from build123d import *

# Parameters (mm, degrees)
IZIM1_W                     = 15
IZIM1_H                     = 15
Y_KSEKLIK_EKSTR_ZYON1_DEPTH = 2
IZIM2_W                     = 2.224225473
IZIM2_H                     = 2
Y_KSEKLIK_EKSTR_ZYON2_DEPTH = 20
Y_KSEKLIK_EKSTR_ZYON3_DEPTH = 2
RADYUS1_R                   = 10
RADYUS2_R                   = 10


with BuildPart() as part:
    # Çizim1 → Yükseklik-Ekstrüzyon1 (new body)
    with BuildSketch(Plane(origin=(0, 0, 0), x_dir=(1, 0, 0), z_dir=(0, 1, 0))):
        Rectangle(IZIM1_W, IZIM1_H)
    extrude(amount=Y_KSEKLIK_EKSTR_ZYON1_DEPTH)

    # Çizim2 → Yükseklik-Ekstrüzyon2 (add)
    with BuildSketch(Plane.XY.offset(7.5)):
        with Locations((1.112112737, 1)):
            Rectangle(IZIM2_W, IZIM2_H)
        with Locations((-1.112112737, 1)):
            Rectangle(IZIM2_W, IZIM2_H)
    extrude(amount=Y_KSEKLIK_EKSTR_ZYON2_DEPTH)

    # Çizim3 → Yükseklik-Ekstrüzyon3 (add)
    with BuildSketch(Plane(origin=(0, 0, 0), x_dir=(1, 0, 0), z_dir=(0, 1, 0))):
        Polygon((-2.224225473, -27.5), (2.224225473, -27.5), (0, -37.5), align=None)
    extrude(amount=Y_KSEKLIK_EKSTR_ZYON3_DEPTH)

    # Radyus1
    radyus1_edges = [part.edges().sort_by_distance(p)[0] for p in [
        (-2.224225473, 1, 27.5),
    ]]
    fillet(radyus1_edges, radius=RADYUS1_R)

    # Radyus2
    radyus2_edges = [part.edges().sort_by_distance(p)[0] for p in [
        (2.224225473, 1, 27.5),
    ]]
    fillet(radyus2_edges, radius=RADYUS2_R)


solid = part.part
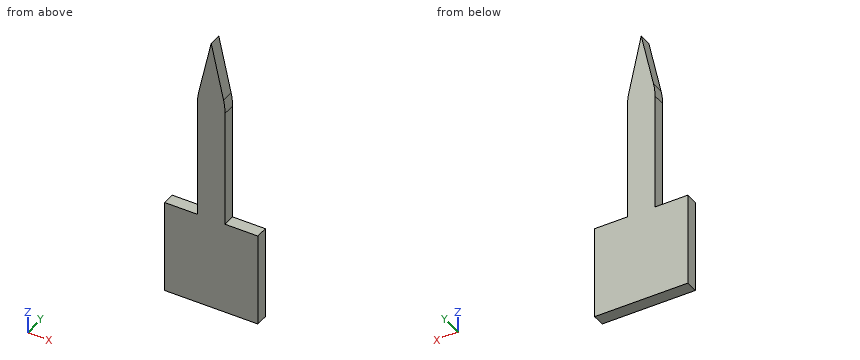
Input: part model. Units: mm. Frame: model coordinates. Round coordinates to 2 decimals unless told otherwise and drop trailing zeros. Write each loop counter-clockwise with the first axis right and the second up, starting at its lowest first coordinate (ties: lowest second). Pieces come first, ordered by that corner, then holes.
1) Ray query, L1, parallel to Z at x = -6, y = 1.45; L2, parallel to X at y = 0.75, z = 9. Return the intervals inside material, ascending.
2) Cut plane A-A (y = 1.6). Return the cut outline in (x, z), then the cut area to 3 significant figures.
3) Cut plane B-B (z = 22.5). Return the cut outline in (x, y), then the cut area to 3 significant figures.
4) Cut plane C-C (x = 6.5). Return the cut outline in (y, z).
5) Contact query for flat-ended pins moving along their axis: P1, Ø1, axis at x = -5.5, y = 1, coming from the +Z side; P2, Ø0.6, axis at y = 1.5, z = 20, coming from the -X side; P3, Ø5, axis at x = 1.5, z = -1.5, coming from the -Y side; P4, Ø1, axis at y = 1, z = 12.5, coming from the +X side. Output: stop coordinate, or through.
Geometry says:
1. L1: z = -7.5 to 7.5
1. L2: x = -2.22 to 2.22
2. outline: (-7.5, -7.5) - (7.5, -7.5) - (7.5, 7.5) - (2.22, 7.5) - (2.22, 26.4) arc R10 ccw to (1.99, 28.57) - (0, 37.5) - (-1.99, 28.57) arc R10 ccw to (-2.22, 26.4) - (-2.22, 7.5) - (-7.5, 7.5) - close
2. area: 336 mm2
3. outline: (-2.22, 0) - (2.22, 0) - (2.22, 2) - (-2.22, 2) - close
3. area: 8.90 mm2
4. outline: (0, -7.5) - (2, -7.5) - (2, 7.5) - (0, 7.5) - close
5. P1: stops at z = 7.5
5. P2: stops at x = -2.22
5. P3: stops at y = 0
5. P4: stops at x = 2.22
